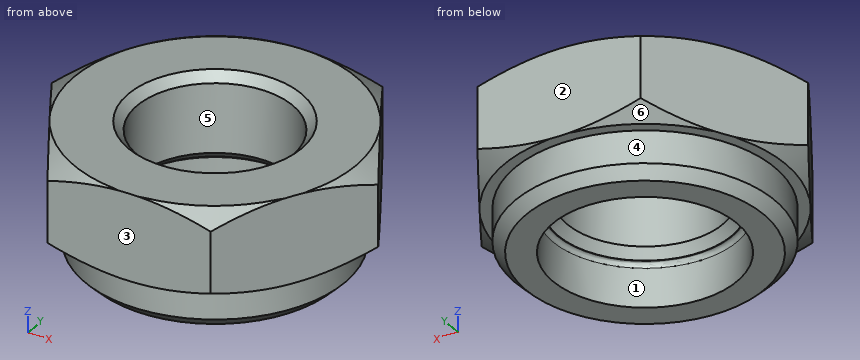
```python
from build123d import *

# Parameters (mm, degrees)
SKETCH3_W          = 26
SKETCH3_H          = 26
CUT_EXTRUDE1_DEPTH = 6


with BuildPart() as part:
    # Sketch1 → Revolve1 (revolve)
    with BuildSketch(Plane(origin=(0, 0, 0), x_dir=(0, 0, -1), z_dir=(1, 0, 0)), mode=Mode.PRIVATE) as revolve1_sk:
        Polygon((-6, 0), (-6, 6.5), (-5.24944465, 7.8), (-2.75055535, 7.8), (-2, 6.5), (-2, 6), (-0.5, 6), (0, 5.5), (0, 0), align=None)
    revolve(revolve1_sk.sketch.rotate(Axis((0, 0, 0), (0, 0, 1)), 270), axis=Axis((0, 0, 0), (0, 0, 1)))

    # Sketch2 → Cut-Revolve1 (revolve, cut)
    with BuildSketch(Plane(origin=(0, 0, 0), x_dir=(0, 0, -1), z_dir=(1, 0, 0)), mode=Mode.PRIVATE) as cut_revolve1_sk:
        with BuildLine():
            Line((-6, 0), (-6, 4))
            Line((-6, 4), (-5.594, 3.594))
            Line((-5.594, 3.594), (-2.406, 3.594))
            Line((-2.406, 3.594), (-2, 4))
            Line((-2, 4), (-2, 4.05))
            ThreePointArc((-2, 4.05), (-1.941421356, 4.191421356), (-1.8, 4.25))
            Line((-1.8, 4.25), (0, 4.25))
            Line((0, 4.25), (0, 0))
            Line((0, 0), (-6, 0))
        make_face()
    revolve(cut_revolve1_sk.sketch.rotate(Axis((0, 0, 0), (0, 0, 1)), 270), axis=Axis((0, 0, 0), (0, 0, 1)), mode=Mode.SUBTRACT)

    # Sketch3 → Cut-Extrude1 (cut)
    with BuildSketch(Plane.XY):
        Rectangle(SKETCH3_W, SKETCH3_H)
        Polygon((-7.505553499, 0), (-3.75277675, -6.5), (3.75277675, -6.5), (7.505553499, 0), (3.75277675, 6.5), (-3.75277675, 6.5), align=None, mode=Mode.SUBTRACT)
    extrude(amount=CUT_EXTRUDE1_DEPTH, mode=Mode.SUBTRACT)


solid = part.part
```
Geometry: final body of the model. Coordinates: model frame, mm. Face numbers are marked on the shaded views. A direction names the side the tool comes from. Coordinates: 2 decimals unless noted, no trailing zeros. Order: outer loops, then holes, each group sorted by start corner. A loop starts at its lowest first (then second) coordinate and runs counter-clockwise, first axis right, second up. Notation, with made-up numbers: (-39, 46) -> (-12, 46) arc R27 ccw to (-12, 82) -> close; hole circle Ø4 at (86, 30.5). An arc over 180 degrees is marked (long way). Answer in a Markdown table with one row per item.
Item 1: Contact query for flat-ended pins moving along their axis: P1, Ø1.5, axis at y = -2, z = 4.5, coming from the -X side; P2, Ø1.5, axis at y = -2, z = 0.5, coming from the +X side. Output: stop coordinate, or through.
Return value:
| item | result |
|---|---|
| P1 | stops at x = -6.78 |
| P2 | stops at x = 5.87 |
Item 2: Draft query along Y for the marked faces 3, 4, 5 and 6. Return one class per face: released by +Y, released by -Y, zero draft, split by the parting line, or undercut.
Return value:
| item | result |
|---|---|
| face 3 | released by -Y |
| face 4 | split by the parting line |
| face 5 | undercut |
| face 6 | released by +Y |
Item 3: Ray query, L1, parallel to Y at x = 0, z = 1.15; L2, parallel to Y at x = 3.25, z = 3.25; L3, parallel to X at y = 3, z = 2.25. Return the intervals inside material, ascending.
Return value:
| item | result |
|---|---|
| L1 | y = -6 to -4.25, 4.25 to 6 |
| L2 | y = -6.5 to -1.53, 1.53 to 6.5 |
| L3 | x = -5.77 to -2.25, 2.25 to 5.77 |
Item 4: Section A-A on z = 3.25. Output: boundary loops of the cut face in (x, y), plus the area to 3 significant figures.
Return value:
| item | result |
|---|---|
| outline | (-7.51, 0) -> (-3.75, -6.5) -> (3.75, -6.5) -> (7.51, 0) -> (3.75, 6.5) -> (-3.75, 6.5) -> close; hole circle Ø7.19 at (0, 0) |
| area | 106 mm² |
Item 5: Section B-B on z = 0.75. Output: boundary loops of the cut face in (x, y).
Return value:
| item | result |
|---|---|
| outline | circle Ø12 at (0, 0); hole circle Ø8.5 at (0, 0) |
Item 6: Access query for the marked faces 1 and 2. Directions: +Z, -Z, +X, -X, +Y, -Y. A direction counts if a zero-diameter tool reaches every point of the face in a straight line with its end or side. Return the directions, or none.
Return value:
| item | result |
|---|---|
| face 1 | -Z |
| face 2 | +Z, -Z, +X, -X, +Y |
